Can you work these out from the model? Positions are in its coordinate system, mm. Face numbers are marked on the shaded views. A direction names the side the tool comes from. Coordinates: 2 decimals unless noted, no trailing zeros. Order: outer loops, then holes, each group sorted by start corner. A loop starts at its lowest first (then second) coordinate and runs counter-clockwise, first axis right, second up.
```python
from build123d import *

# Parameters (mm, degrees)
SKETCH1_R           = 29
BOSS_EXTRUDE2_DEPTH = 5
SKETCH3_R           = 10.5
BOSS_EXTRUDE3_DEPTH = 8
SKETCH4_R           = 3
CUT_EXTRUDE1_DEPTH  = 44.023249529
SKETCH6_R           = 10
BOSS_EXTRUDE5_DEPTH = 7
SKETCH8_R           = 3
CUT_EXTRUDE3_DEPTH  = 44.023249529
SKETCH9_R           = 2.5
CUT_EXTRUDE4_DEPTH  = 43.731721238
SKETCH10_R          = 4.5
CUT_EXTRUDE5_DEPTH  = 43.731721238


with BuildPart() as part:
    # Sketch1 → Boss-Extrude2 (new body)
    with BuildSketch(Plane(origin=(0, 0, 0), x_dir=(1, 0, 0), z_dir=(0, 1, 0))):
        with Locations(Location((0, 0, 0), (0, 0, 270))):
            Circle(SKETCH1_R)
    extrude(amount=BOSS_EXTRUDE2_DEPTH)

    # Sketch3 → Boss-Extrude3 (add)
    with BuildSketch(Plane(origin=(0, 5, 0), x_dir=(1, 0, 0), z_dir=(0, 1, 0))):
        with Locations(Location((0, 0, 0), (0, 0, 270))):
            Circle(SKETCH3_R)
    extrude(amount=BOSS_EXTRUDE3_DEPTH)

    # Sketch4 → Cut-Extrude1 (cut, through all)
    with BuildSketch(Plane(origin=(0, 13, 0), x_dir=(1, 0, 0), z_dir=(0, 1, 0))):
        with Locations(Location((0, 0, 0), (0, 0, 270))):
            Circle(SKETCH4_R)
    extrude(amount=-CUT_EXTRUDE1_DEPTH, mode=Mode.SUBTRACT)

    # Sketch6 → Boss-Extrude5 (add)
    with BuildSketch(Plane.XZ):
        with Locations(Location((0, 0, 0), (0, 0, 90))):
            Circle(SKETCH6_R)
    extrude(amount=BOSS_EXTRUDE5_DEPTH)

    # Sketch8 → Cut-Extrude3 (cut, through all)
    with BuildSketch(Plane(origin=(0, 0, 0), x_dir=(1, 0, 0), z_dir=(0, 1, 0))):
        with Locations(Location((0, 0, 0), (0, 0, 270))):
            Circle(SKETCH8_R)
    extrude(amount=-CUT_EXTRUDE3_DEPTH, mode=Mode.SUBTRACT)

    # Sketch9 → Cut-Extrude4 (cut, through all)
    with BuildSketch(Plane(origin=(0, 5, 0), x_dir=(1, 0, 0), z_dir=(0, 1, 0))):
        with Locations(Location((11.5, 19.918584287, 0), (0, 0, 270))):
            Circle(SKETCH9_R)
        with Locations(Location((-23, 0, 0), (0, 0, 270))):
            Circle(SKETCH9_R)
        with Locations(Location((11.5, -19.918584287, 0), (0, 0, 270))):
            Circle(SKETCH9_R)
    extrude(amount=-CUT_EXTRUDE4_DEPTH, mode=Mode.SUBTRACT)

    # Sketch10 → Cut-Extrude5 (cut, through all)
    with BuildSketch(Plane(origin=(0, 5, 0), x_dir=(1, 0, 0), z_dir=(0, 1, 0))):
        with Locations(Location((-11.5, -19.918584287, 0), (0, 0, 270))):
            Circle(SKETCH10_R)
        with Locations(Location((-11.5, 19.918584287, 0), (0, 0, 270))):
            Circle(SKETCH10_R)
        with Locations(Location((23, 0, 0), (0, 0, 270))):
            Circle(SKETCH10_R)
    extrude(amount=-CUT_EXTRUDE5_DEPTH, mode=Mode.SUBTRACT)


solid = part.part
```
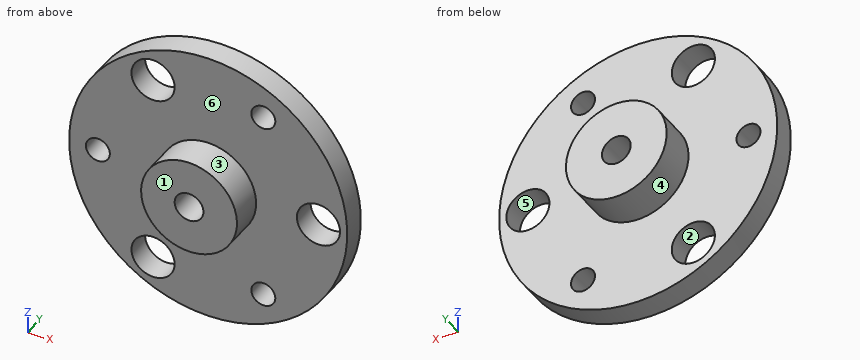
1. Thinking about a two-plate mould opening in Z: for the marked faces 1, 2 and 3, which applies, pulls with the +Z half, pulls with the -Z half, needs draft (parallel to the pull), parting line crosses it, or undercut?
Completed:
face 1: needs draft
face 2: undercut
face 3: parting line crosses it
2. Imagine slicing it at D-D on x = -11.5. Please give me the cut outline in (y, z), then the cut area to 3 significant figures.
Completed:
outline: (0, -26.62) - (5, -26.62) - (5, -24.42) - (0, -24.42) - close; (0, -15.42) - (5, -15.42) - (5, 15.42) - (0, 15.42) - close; (0, 24.42) - (5, 24.42) - (5, 26.62) - (0, 26.62) - close
area: 176 mm2
3. Imagine slicing it at B-B on x = 1. Please give me the cut outline in (y, z).
Completed:
outline: (-7, -9.95) - (0, -9.95) - (0, -28.98) - (5, -28.98) - (5, -10.45) - (13, -10.45) - (13, -2.83) - (-7, -2.83) - close; (-7, 2.83) - (13, 2.83) - (13, 10.45) - (5, 10.45) - (5, 28.98) - (0, 28.98) - (0, 9.95) - (-7, 9.95) - close
4. Imagine slicing it at A-A on z = 0. Please give me the cut outline in (x, y), then the cut area to 3 significant figures.
Completed:
outline: (-29, 0) - (-25.5, 0) - (-25.5, 5) - (-29, 5) - close; (-20.5, 0) - (-10, 0) - (-10, -7) - (-3, -7) - (-3, 13) - (-10.5, 13) - (-10.5, 5) - (-20.5, 5) - close; (3, -7) - (10, -7) - (10, 0) - (18.5, 0) - (18.5, 5) - (10.5, 5) - (10.5, 13) - (3, 13) - close; (27.5, 0) - (29, 0) - (29, 5) - (27.5, 5) - close
area: 408 mm2
5. I'm going to push flat-ended pins straight in: pin 1 (10 mm diameter, centred on y = 4, z = 3.5, fed in from -X); pin 2 (4 mm diameter, centred on y = 4, z = 10, fed in from -X); pin 3 (6 mm diameter, centred on x = -0.5, z = -19.5, fed in from +Y); pin 4 (5.5 mm diameter, centred on x = 23, z = 0, fed in from -Y). Where does each tip first touch, or does it pass through?
Completed:
pin 1: stops at x = -29
pin 2: stops at x = -27.87
pin 3: stops at y = 5
pin 4: passes through
6. Please list where these lines run through material, in increasing order: probe 1 along X at (y, z) = (1.5, 0); probe 2 along X at (y, z) = (-1.5, 0); probe 3 along Y at (x, z) = (5, 24.5).
Completed:
probe 1: x = -29 to -25.5, -20.5 to -3, 3 to 18.5, 27.5 to 29
probe 2: x = -10 to -3, 3 to 10
probe 3: y = 0 to 5
7. On a 3-axis mill with a long thin cutter (end or side, diameter ignored), from which of +Z, -Z, +X, -X, +Y, -Y can I reach the whole of each face in a straight line? I mean the marked faces 4, 5 and 6. Say none if no direction works.
Completed:
face 4: +Y
face 5: +Y, -Y
face 6: -Y
8. Imagine slicing it at C-C on z = -23.5. Please give me the cut outline in (x, y), then the cut area to 3 significant figures.
Completed:
outline: (-16.99, 0) - (-14.22, 0) - (-14.22, 5) - (-16.99, 5) - close; (-8.78, 0) - (16.99, 0) - (16.99, 5) - (-8.78, 5) - close
area: 143 mm2
